from build123d import *

# Parameters (mm, degrees)
SKETCH1_R               = 22.5
BOSS_EXTRUDE1_DEPTH     = 5
SKETCH2_R               = 13
BOSS_EXTRUDE2_DEPTH     = 9.2
BOSS_EXTRUDE4_START     = 5
SKETCH5_R               = 22.5
BOSS_EXTRUDE4_DEPTH     = 5
SKETCH6_R               = 4
SKETCH6_R_2             = 1.85
CUT_EXTRUDE1_DEPTH      = 38.163691959
FILLET1_R               = 5
CUT_EXTRUDE2_DEPTH      = 26
CUT_EXTRUDE2_DEPTH_BACK = 26
SKETCH8_R               = 1.85


with BuildPart() as part:
    # Sketch1 → Boss-Extrude1 (new body)
    with BuildSketch(Plane.XY):
        Circle(SKETCH1_R)
    extrude(amount=BOSS_EXTRUDE1_DEPTH)

    # Sketch2 → Boss-Extrude2 (add)
    with BuildSketch(Plane.XY):
        Circle(SKETCH2_R)
    extrude(amount=-BOSS_EXTRUDE2_DEPTH)

    # Sketch5 → Boss-Extrude4 (add)
    with BuildSketch(Plane(origin=(0, 0, -9.2), x_dir=(-1, 0, 0), z_dir=(0, 0, -1)).offset(BOSS_EXTRUDE4_START)):
        with Locations(Location((0, 0, 0), (0, 0, 180))):
            Circle(SKETCH5_R)
    extrude(amount=-BOSS_EXTRUDE4_DEPTH)

    # Sketch6 → Cut-Extrude1 (cut, through all)
    with BuildSketch(Plane.XY.offset(5)):
        Circle(SKETCH6_R)
        with Locations((0, 8)):
            Circle(SKETCH6_R_2)
        with Locations((8, 0)):
            Circle(SKETCH6_R_2)
        with Locations((0, -8)):
            Circle(SKETCH6_R_2)
        with Locations((-8, 0)):
            Circle(SKETCH6_R_2)
    extrude(amount=-CUT_EXTRUDE1_DEPTH, mode=Mode.SUBTRACT)

    # Fillet1
    fillet1_edges = [part.edges().sort_by_distance(p)[0] for p in [
        (-22.5, 0, 0),
        (-22.5, 0, -9.2),
    ]]
    fillet(fillet1_edges, radius=FILLET1_R - 0.0001)  # a hair under: the kernel refuses the full size

    # Sketch8 → Cut-Extrude2 (cut, two sides: drawn at the far end of the back side and taken through both)
    with BuildSketch(Plane(origin=(0, 0, 0), x_dir=(1, 0, 0), z_dir=(0, 1, 0)).offset(-CUT_EXTRUDE2_DEPTH_BACK)):
        with Locations(Location((0, 4.5, 0), (0, 0, 90))):
            Circle(SKETCH8_R)
    extrude(amount=CUT_EXTRUDE2_DEPTH + CUT_EXTRUDE2_DEPTH_BACK, mode=Mode.SUBTRACT)


solid = part.part
Geometry: final body of the model. Coordinates: model frame, mm. A direction names the side the tool comes from. Give positions to 0.01 mm unless a question says otherwise; leave off trailing zeros. Loops run counter-clockwise (first coordinate to the right, second up) from the corner with the lowest first, then second, coordinate; pieces in that order, holes last. Notation, with made-up numbers: (17.5, 64) - (26.5, 64) arc R18 ccw to (26.5, 90) - close; hole circle Ø2 at (47.5, 36). An arc over 180 degrees is marked (long way). One line per question, with ' | ' between items. Start each with the question number.
(1) Ray query, line 1 (Y direction, x = 0, z = -2); line 2 (Z direction, x = 3, y = -13); line 3 (Y direction, x = -1.5, z = -1.75). Return the intervals inside material, ascending. Write a range as from..to.
(2) Reachability of faces 1 (the flat face through (-3, -13, -9.2)), 2 (the cylindrical face through (6.15, 0.08, -4.47)) from +Z, -Z, +X, -X, +Y, -Y: full face, straight path, thin tool, end or side. Return the list, or none.
(3) Section query B-B on z = -7.75. Return loops of the section in (x, y).
(4) Section query D-D on z = -12.5. Return loops of the section in (x, y).
(5) Pull-direction query (X, two-part tool) for faces 3 (the flat face through (-3, 13, 0)), 4 (the cylindrical face through (-1.85, -7.92, -10.36)), 5 (the cylindrical face through (-2.82, -12.69, -4.54)); classes: released by +X, released by -X, zero draft, split by the parting line, or undercut.
(6) Section query A-A on y = 0. Count the separate pieces of the cut face and the enclosed holes in it, then the cut area to 3 significant figures.
(7) Contact query for flat-ended pins moving along their axis: pin 1 (6 mm diameter, centred on y = -2.5, z = 0.5, fed in from +X); pin 2 (3.5 mm diameter, centred on x = 0, z = -4.5, fed in from +Y); pin 3 (5 mm diameter, centred on x = 8, y = 0, fed in from +Z); pin 4 (4 mm diameter, centred on x = -3, z = -11, fed in from -Y). Output: stop coordinate, or through.
The answers:
1) line 1: -13..-9.85, -6.15..-4, 4..6.15, 9.85..13 | line 2: -14.2..-9.2, 0..5 | line 3: -12.91..-9.08, -6.92..-3.71, 3.71..6.92, 9.08..12.91
2) face 1: none | face 2: +Z, -Z
3) outline: circle Ø26 at (0, 0); hole circle Ø3.7 at (-8, 0); hole circle Ø8 at (0, 0); hole circle Ø3.7 at (0, -8); hole circle Ø3.7 at (0, 8); hole circle Ø3.7 at (8, 0)
4) outline: circle Ø44.4 at (0, 0); hole circle Ø3.7 at (-8, 0); hole circle Ø8 at (0, 0); hole circle Ø3.7 at (0, -8); hole circle Ø3.7 at (0, 8); hole circle Ø3.7 at (8, 0)
5) face 3: zero draft | face 4: undercut | face 5: split by the parting line
6) separate pieces: 4 | enclosed holes: 0 | area: 372 mm2
7) pin 1: x = 22.17 | pin 2: through | pin 3: z = 5 | pin 4: y = -22.2
